Geometry: see drawing. Coordinates: mm, zero at the bounding-box minimum. A direction names the side the tool comes from. Give positions to 0.01 mm unless a question says otherwise; leave off trailing zeros. Loops run counter-clockwise (first coordinate to the right, second up) from the corner with the lowest first, then second, coordinate; pieces in that order, holes last. Notation, with made-up numbers: (78, 45.5) -> (135, 45.5) arc R9 cw to (135, 57.5) -> close; hole circle Ø9 at (71.25, 56.25). An arc over 180 degrees is marked (long way). Return JSON: item names as keys, results as strings. Group by question number.
(1) Cut plane B-B on y = 24.5. Return loops of the section in (x, z).
(2) Draft query along X for the marked faces 3, 4, 5 and 6. Return one class per face: released by +X, released by -X, zero draft, split by the parting line, or undercut.
(3) Cut plane C-C on x = 25. Return loops of the section in (y, z).
(4) Pin query (flat end, axial travel): pin 1 (8 mm diameter, centred on x = 8.5, z = 5, fed in from +Y); pin 2 (4.5 mm diameter, centred on y = 10, z = 10, fed in from +X). Return the tip coordinate at first contact, or that it passes through.
(5) Cut plane D-D on z = 10. Return loops of the section in (x, y).
(6) Access query for the marked faces 1 and 2. Directions: +Z, -Z, +X, -X, +Y, -Y. A direction counts if a zero-diameter tool reaches every point of the face in a straight line with its end or side. Return the directions, or none.
(7) Cut plane A-A on z = 15. Return loops of the section in (x, y), then the cut area to 3 significant figures.
(8) Ray query, line 1 (X direction, y = 15.25, z = 4.25); line 2 (Z direction, x = 49.3, y = 10); line 3 (Y direction, x = 7, z = 15.25). Return the intervals inside material, ascending. Write a range as from..to.
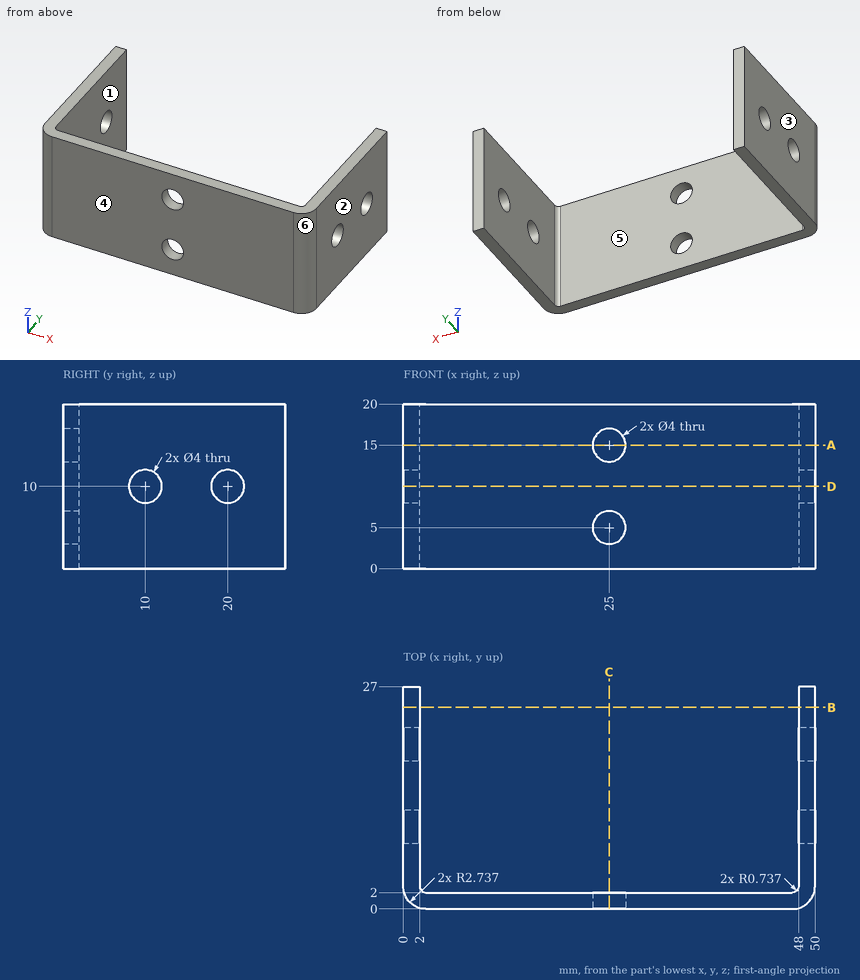
Answers:
{
 "1": {"outline": "(0, 0) -> (2, 0) -> (2, 20) -> (0, 20) -> close; (48, 0) -> (50, 0) -> (50, 20) -> (48, 20) -> close"},
 "2": {"face 3": "released by -X", "face 4": "zero draft", "face 5": "undercut", "face 6": "released by +X"},
 "3": {"outline": "(0, 0) -> (2, 0) -> (2, 3) -> (0, 3) -> close; (0, 7) -> (2, 7) -> (2, 13) -> (0, 13) -> close; (0, 17) -> (2, 17) -> (2, 20) -> (0, 20) -> close"},
 "4": {"pin 1": "y = 2", "pin 2": "x = 50"},
 "5": {"outline": "(0, 2.74) arc R2.74 ccw to (2.74, 0) -> (47.26, 0) arc R2.74 ccw to (50, 2.74) -> (50, 8) -> (48, 8) -> (48, 2.74) arc R0.74 cw to (47.26, 2) -> (2.74, 2) arc R0.74 cw to (2, 2.74) -> (2, 8) -> (0, 8) -> close; (0, 12) -> (2, 12) -> (2, 18) -> (0, 18) -> close; (0, 22) -> (2, 22) -> (2, 27) -> (0, 27) -> close; (48, 12) -> (50, 12) -> (50, 18) -> (48, 18) -> close; (48, 22) -> (50, 22) -> (50, 27) -> (48, 27) -> close"},
 "6": {"face 1": "+Z, -Z, +Y", "face 2": "+Z, -Z, +X, +Y, -Y"},
 "7": {"outline": "(0, 2.74) arc R2.74 ccw to (2.74, 0) -> (23, 0) -> (23, 2) -> (2.74, 2) arc R0.74 cw to (2, 2.74) -> (2, 27) -> (0, 27) -> close; (27, 0) -> (47.26, 0) arc R2.74 ccw to (50, 2.74) -> (50, 27) -> (48, 27) -> (48, 2.74) arc R0.74 cw to (47.26, 2) -> (27, 2) -> close", "area": "189 mm²"},
 "8": {"line 1": "0..2, 48..50", "line 2": "0..8, 12..20", "line 3": "0..2"}
}
